from build123d import *

# Parameters (mm, degrees)
F1_DEPTH = 101.6
F2_T     = -6.35
F3_W     = 88.9
F3_H     = 6.35
F4_DEPTH = 95.25
F5_R     = 3.81
F6_DEPTH = 25.4


with BuildPart() as f1:
    # F0 (on Front) → F1 (new body)
    with BuildSketch(Plane.XZ):
        Polygon((0, 0), (0, 152.4), (-101.6, 152.4), (-101.6, 0), (-101.6, -76.2), (101.6, -76.2), (101.6, 0), align=None)
    extrude(amount=F1_DEPTH)

    # F2
    f2_openings = [f1.faces().sort_by_distance(p)[0] for p in [
        (-50.8, -50.8, 152.4),
        (-25.4, 0, 19.05),
        (0, -50.8, -76.2),
    ]]
    offset(amount=F2_T, openings=f2_openings, kind=Kind.INTERSECTION)

    # F3 (on face) → F4 (join)
    with BuildSketch(Plane(origin=(0, -95.25, 0), x_dir=(-1, 0, 0), z_dir=(0, 1, 0))):
        with Locations((50.8, -3.175)):
            Rectangle(F3_W, F3_H)
    extrude(amount=F4_DEPTH)

    # F5 (on face) → F6 (cut)
    with BuildSketch(Plane.XZ.offset(101.6)):
        with Locations((-76.2, -63.5)):
            Circle(F5_R)
        with Locations((25.4, -63.5)):
            Circle(F5_R)
    extrude(amount=-F6_DEPTH, mode=Mode.SUBTRACT)

    # F7: F1 across face


with BuildPart() as f1_1:
    add(f1.part)
    add(f1.part.mirror(Plane(origin=(-23.9058823529, 0, 25.9602941176), x_dir=(1, 0, 0), z_dir=(0, 1, 0))))


solid = f1_1.part
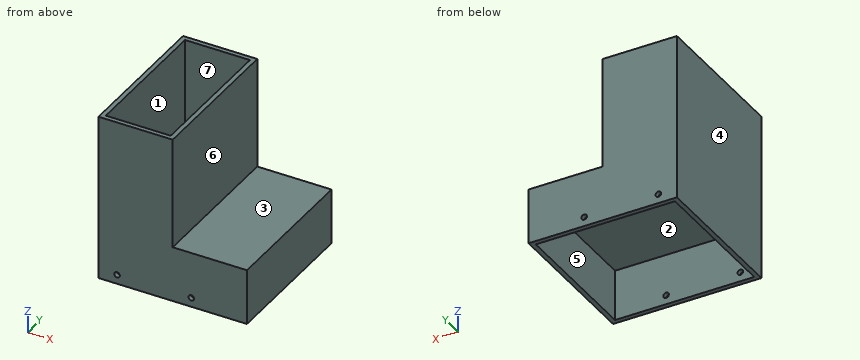
Part model, mm, in its own coordinate system. Face numbers are marked on the shaded views. A direction names the side the tool comes from. Round coordinates to 2 decimals unless told otherwise and drop trailing zeros. Order: outer loops, then holes, each group sorted by start corner. A loop starts at its lowest first (then second) coordinate and runs counter-clockwise, first axis right, second up. Notation, with made-up numbers: (-38, 56.5) -> (14, 56.5) arc R8 cw to (14, 70.5) -> close; hole circle Ø10 at (72.5, -16). An arc over 180 degrees is marked (long way). Put each result on its own line as item: value.
Q1. Band-saw the part on C-C (y = -75.5). Give the cut face in (x, z), and give its area (3 significant figures).
From the geometry:
outline: (-101.6, -76.2) -> (-95.25, -76.2) -> (-95.25, -6.35) -> (95.25, -6.35) -> (95.25, -76.2) -> (101.6, -76.2) -> (101.6, 0) -> (0, 0) -> (0, 152.4) -> (-6.35, 152.4) -> (-6.35, 0) -> (-95.25, 0) -> (-95.25, 152.4) -> (-101.6, 152.4) -> close
area: 4,110 mm2
Q2. Pull direction X, two halves, no side cores. Call the marked faces 4, 5, 6 and 7: pulls with the +X half, pulls with the -X half, needs draft (parallel to the pull), parting line crosses it, or undercut.
From the geometry:
face 4: pulls with the -X half
face 5: undercut
face 6: pulls with the +X half
face 7: undercut
Q3. Band-saw the part on D-D (z = -63.5). Give the cut face in (x, y).
From the geometry:
outline: (-101.6, -101.6) -> (-80.01, -101.6) -> (-80.01, -95.25) -> (-95.25, -95.25) -> (-95.25, 95.25) -> (-80.01, 95.25) -> (-80.01, 101.6) -> (-101.6, 101.6) -> close; (-72.39, -101.6) -> (21.59, -101.6) -> (21.59, -95.25) -> (-72.39, -95.25) -> close; (-72.39, 95.25) -> (21.59, 95.25) -> (21.59, 101.6) -> (-72.39, 101.6) -> close; (29.21, -101.6) -> (101.6, -101.6) -> (101.6, 101.6) -> (29.21, 101.6) -> (29.21, 95.25) -> (95.25, 95.25) -> (95.25, -95.25) -> (29.21, -95.25) -> close
Q4. Band-saw the part on B-B (z = -19.5). Give the cut face in (x, y).
From the geometry:
outline: (-101.6, -101.6) -> (101.6, -101.6) -> (101.6, 101.6) -> (-101.6, 101.6) -> close; hole (-95.25, -95.25) -> (95.25, -95.25) -> (95.25, 95.25) -> (-95.25, 95.25) -> close
Q5. Band-saw the part on A-A (x = -76.2). Give the cut face in (y, z).
From the geometry:
outline: (-101.6, -76.2) -> (-95.25, -76.2) -> (-95.25, -67.31) -> (-101.6, -67.31) -> close; (-101.6, -59.69) -> (-95.25, -59.69) -> (-95.25, -6.35) -> (95.25, -6.35) -> (95.25, -59.69) -> (101.6, -59.69) -> (101.6, 152.4) -> (95.25, 152.4) -> (95.25, 0) -> (-95.25, 0) -> (-95.25, 152.4) -> (-101.6, 152.4) -> close; (95.25, -76.2) -> (101.6, -76.2) -> (101.6, -67.31) -> (95.25, -67.31) -> close
Q6. Wall check: line 1 (X direction, y = 99, z = -63); line 2 (X direction, y = 71, z = 92.5); line 3 (X direction, y = -62.5, z = -34.5). Give the ranges that are in metal, low to high. Write a range as [from, to].
From the geometry:
line 1: x = [-101.6, -79.98], [-72.42, 21.62], [29.18, 101.6]
line 2: x = [-101.6, -95.25], [-6.35, 0]
line 3: x = [-101.6, -95.25], [95.25, 101.6]
Q7. Pin check, flat tips, straight feed: pin 1 Ø1 at (x, y) = (59, 18.5) entering from -Z; pin 2 Ø5 at (x, y) = (-60.5, -28) entering from +Z; pin 3 Ø5 at (y, z) = (71, 16.5) entering from +X; pin 4 Ø6 at (x, z) = (-76.2, -63.5) entering from -Y. Stop position of each tip, or through.
From the geometry:
pin 1: stops at z = -6.35
pin 2: stops at z = 0
pin 3: stops at x = 0
pin 4: passes through
Q8. Tool access for the marked faces 1, 2 and 3: list every direction of +Z, -Z, +X, -X, +Y, -Y with a clear straight run to the whole face (end or side of a thin tool).
From the geometry:
face 1: +Z
face 2: -Z
face 3: +Z, +X, +Y, -Y
